from build123d import *

# Parameters (mm, degrees)
F1_DEPTH = 34.544
F3_DEPTH = 7.874
F5_DEPTH = 9.652
F6_R     = 7.112
F7_DEPTH = 25.4
F8_R     = 6.35


with BuildPart() as f1:
    # F0 (on Front) → F1 (new body)
    with BuildSketch(Plane.XZ):
        Polygon((0, 0), (0, 25.4), (-9.652, 25.4), (-9.652, 7.874), (-76.2, 7.874), (-76.2, 47.752), (-84.074, 47.752), (-84.074, 0), align=None)
    extrude(amount=F1_DEPTH)

    # F2 (on face) → F3 (join)
    with BuildSketch(Plane(origin=(-84.074, 0, 0), x_dir=(0, -1, 0), z_dir=(-1, 0, 0))):
        with BuildLine():
            ThreePointArc((34.544, 47.752), (17.272, 65.024), (0, 47.752))
            Line((0, 47.752), (34.544, 47.752))
        make_face()
    extrude(amount=-F3_DEPTH)

    # F4 (on face) → F5 (join)
    with BuildSketch(Plane.YZ):
        with BuildLine():
            Line((6.8788736876, 65.024), (-17.272, 65.024))
            Line((-17.272, 65.024), (-43.2572502127, 65.024))
            ThreePointArc((-43.2572502127, 65.024), (-60.480665025, 46.4574088668), (-40.6753511738, 30.6740674157))
            ThreePointArc((-40.6753511738, 30.6740674157), (-36.3996034701, 29.4437993991), (-34.544, 25.4))
            Line((-34.544, 25.4), (0, 25.4))
            ThreePointArc((0, 25.4), (2.1892001539, 29.708339579), (6.9598012479, 30.4801895932))
            ThreePointArc((6.9598012479, 30.4801895932), (24.1508262893, 47.7924638912), (6.8788736876, 65.024))
        make_face()
        with BuildLine():
            Line((5.08, 44.196), (-39.624, 44.196))
            ThreePointArc((-39.624, 44.196), (-43.18, 47.752), (-39.624, 51.308))
            Line((-39.624, 51.308), (-34.1739776358, 51.308))
            ThreePointArc((-34.1739776358, 51.308), (-28.1555369251, 61.163584843), (-17.272, 65.024))
            ThreePointArc((-17.272, 65.024), (-6.3884630749, 61.163584843), (-0.3700223642, 51.308))
            Line((-0.3700223642, 51.308), (5.08, 51.308))
            ThreePointArc((5.08, 51.308), (8.636, 47.752), (5.08, 44.196))
        make_face(mode=Mode.SUBTRACT)
        with BuildLine():
            ThreePointArc((-17.272, 65.024), (-28.1555369251, 61.163584843), (-34.1739776358, 51.308))
            Line((-34.1739776358, 51.308), (-0.3700223642, 51.308))
            ThreePointArc((-0.3700223642, 51.308), (-6.3884630749, 61.163584843), (-17.272, 65.024))
        make_face()
    extrude(amount=-F5_DEPTH)

    # F6 (on face) → F7 (cut)
    with BuildSketch(Plane(origin=(-84.074, 0, 0), x_dir=(0, -1, 0), z_dir=(-1, 0, 0))):
        with Locations((17.272, 47.752)):
            Circle(F6_R)
        with Locations((17.272, 28.702)):
            Circle(F6_R)
    extrude(amount=-F7_DEPTH, mode=Mode.SUBTRACT)

    # F8
    f8_edges = [f1.edges().sort_by_distance(p)[0] for p in [
        (-9.652, -17.272, 7.874),
        (-76.2, -17.272, 7.874),
    ]]
    fillet(f8_edges, radius=F8_R)


solid = f1.part
The model under review builds one solid part; all positions refer to its coordinate system, in mm. A direction names the side the tool comes from. Coordinates: 2 decimals unless noted, no trailing zeros. Write each loop counter-clockwise with the first axis right and the second up, starting at its lowest first coordinate (ties: lowest second). Pieces come first, ordered by that corner, then holes. Notation, with made-up numbers: (37, 62.5) -> (65, 62.5) arc R27 ccw to (65, 92.5) -> close; hole circle Ø4 at (-3, 77.5). An arc over 180 degrees is marked (long way). Answer in a Markdown table with one row per item.
1. We need section D-D, the plane x = -42. State the section outline as (y, z) points.
Answers below:
| item | result |
|---|---|
| outline | (-34.54, 0) -> (0, 0) -> (0, 7.87) -> (-34.54, 7.87) -> close |
2. Wall thickness on probe 1 along Z at (x, y) = (-5, -13); probe 2 along X at (y, z) = (-9, 21.5); probe 3 along Z at (x, y) = (-55, -12): over which ranges is each line inside the solid? List them lowest first. Write a range as [from, to].
Answers below:
| item | result |
|---|---|
| probe 1 | z = [0, 44.2], [51.31, 65.02] |
| probe 2 | x = [-84.07, -76.2], [-9.65, 0] |
| probe 3 | z = [0, 7.87] |
3. We need section A-A, the plane z = 38.5. State the section outline as (x, y) points, and give its area (3 significant figures).
Answers below:
| item | result |
|---|---|
| outline | (-84.07, -34.54) -> (-76.2, -34.54) -> (-76.2, 0) -> (-84.07, 0) -> close; (-9.65, -57.84) -> (0, -57.84) -> (0, 21.46) -> (-9.65, 21.46) -> close |
| area | 1,040 mm^2 |
4. For faces 5 (the cylindrical face through (-11.463, -17.514, 9.784)), 6 (the cylindrical face through (-4.758, 8.635, 47.83)), 7 (the flat face through (-5, -17, 44.196)), 8 (the cylindrical face through (-80.192, -10.167, 48.065)), list the 3-axis set-ups (+Z, -Z, +X, -X, +Y, -Y) from which the entire face can be reached by the end or side of a thin tool; tool diameter is ignored.
Answers below:
| item | result |
|---|---|
| face 5 | +Z, +Y, -Y |
| face 6 | +X, -X |
| face 7 | +X |
| face 8 | -X |
5. We need section B-B, the plane y = -42. State the section outline as (x, z) points, and give its area (3 significant figures).
Answers below:
| item | result |
|---|---|
| outline | (-9.65, 30.53) -> (0, 30.53) -> (0, 45.11) -> (-9.65, 45.11) -> close; (-9.65, 50.4) -> (0, 50.4) -> (0, 65.02) -> (-9.65, 65.02) -> close |
| area | 282 mm^2 |
6. Draft analysis for pull direction X (two halves, no side actions). For faces 1 (the cylindrical face through (-80.19, -17.65, 65.02)), 2 (the flat face through (-84.074, -9, 33)), 3 (the flat face through (0, -19, 40)), 4 (the cylindrical face through (-74.29, -17.514, 9.685)), state which applies: +X half, -X half, draft (parallel to the pull), parting line (faces both ways), or undercut.
Answers below:
| item | result |
|---|---|
| face 1 | draft |
| face 2 | -X half |
| face 3 | +X half |
| face 4 | undercut |
7. Clearance check with flat-ended pins moving along their axes: pin 1 Ø17.5 at (x, y) = (-54, -24) entering from +Z; pin 2 Ø12 at (x, z) = (-72, 27.5) entering from -Y; pin 3 Ø4 at (y, z) = (-48.5, 50) entering from -X. State where each tip first meets the part, or that it passes through.
Answers below:
| item | result |
|---|---|
| pin 1 | stops at z = 7.87 |
| pin 2 | stops at y = -34.54 |
| pin 3 | stops at x = -9.65 |
8. We need section C-C, the plane y = -22. State the section outline as (x, z) points.
Answers below:
| item | result |
|---|---|
| outline | (-84.07, 0) -> (0, 0) -> (0, 44.2) -> (-9.65, 44.2) -> (-9.65, 14.22) arc R6.35 cw to (-16, 7.87) -> (-69.85, 7.87) arc R6.35 cw to (-76.2, 14.22) -> (-76.2, 23.39) -> (-84.07, 23.39) -> close; (-84.07, 34.01) -> (-76.2, 34.01) -> (-76.2, 42.44) -> (-84.07, 42.44) -> close; (-84.07, 53.06) -> (-76.2, 53.06) -> (-76.2, 64.36) -> (-84.07, 64.36) -> close; (-9.65, 51.31) -> (0, 51.31) -> (0, 65.02) -> (-9.65, 65.02) -> close |
